from build123d import *

# Parameters (mm, degrees)
SKETCH1_W           = 103
SKETCH1_H           = 115
BOSS_EXTRUDE2_DEPTH = 20
SKETCH3_W           = 21
SKETCH3_H           = 25
CUT_EXTRUDE1_DEPTH  = 10
CUT_EXTRUDE2_DEPTH  = 46


with BuildPart() as part:
    # Sketch1 → Boss-Extrude2 (new body)
    with BuildSketch(Plane.XY):
        with Locations((51.5, 57.5)):
            Rectangle(SKETCH1_W, SKETCH1_H)
    extrude(amount=BOSS_EXTRUDE2_DEPTH)

    # Sketch3 → Cut-Extrude1 (cut)
    with BuildSketch(Plane.XY.offset(20)):
        with Locations((20.5, 92.5)):
            Rectangle(SKETCH3_W, SKETCH3_H)
        with Locations((51.5, 92.5)):
            Rectangle(SKETCH3_W, SKETCH3_H)
        with Locations((82.5, 92.5)):
            Rectangle(SKETCH3_W, SKETCH3_H)
        Polygon((10, 70), (10, 54.37934433), (10, 45), (31, 45), (31, 70), align=None)
        with Locations((51.5, 57.5)):
            Rectangle(SKETCH3_W, SKETCH3_H)
        Polygon((10, 35), (10, 17.462651727), (10, 10), (31, 10), (31, 35), align=None)
        with Locations((51.5, 22.5)):
            Rectangle(SKETCH3_W, SKETCH3_H)
        with Locations((82.5, 22.5)):
            Rectangle(SKETCH3_W, SKETCH3_H)
        with Locations((82.5, 57.5)):
            Rectangle(SKETCH3_W, SKETCH3_H)
    extrude(amount=-CUT_EXTRUDE1_DEPTH, mode=Mode.SUBTRACT)

    # Sketch4 → Cut-Extrude2 (cut)
    with BuildSketch(Plane.XY.offset(20)):
        with BuildLine():
            Line((0, 105), (0, 115))
            Line((0, 115), (10, 115))
            ThreePointArc((10, 115), (2.928932188, 112.071067812), (0, 105))
        make_face()
        with BuildLine():
            Line((93, 115), (103, 115))
            Line((103, 115), (103, 105))
            ThreePointArc((103, 105), (100.071067812, 112.071067812), (93, 115))
        make_face()
        with BuildLine():
            Line((103, 10), (103, 0))
            Line((103, 0), (93, 0))
            ThreePointArc((93, 0), (100.071067812, 2.928932188), (103, 10))
        make_face()
        with BuildLine():
            Line((10, 0), (0, 0))
            Line((0, 0), (0, 10))
            ThreePointArc((0, 10), (2.928932188, 2.928932188), (10, 0))
        make_face()
    extrude(amount=-CUT_EXTRUDE2_DEPTH, mode=Mode.SUBTRACT)


solid = part.part
Can you work these out from the model? Positions are in its coordinate system, mm. A direction names the side the tool comes from. Give positions to 0.01 mm unless a question says otherwise; leave off trailing zeros. Loops run counter-clockwise (first coordinate to the right, second up) from the corner with the lowest first, then second, coordinate; pieces in that order, holes last. Notation, with made-up numbers: (5, 11) -> (11, 11) arc R25 cw to (11, 24) -> close; hole circle Ø5 at (0, 35). An arc over 180 degrees is marked (long way). Return JSON: item names as keys, results as strings.
Q1. We'd pull the mould along Y, two halves only. Please class faces 1 (the face through (62, 22, 15)), 2 (the face through (99.99, 2.85, 10.14)), 3 (the face through (51, 58, 0)): released by +Y, released by -Y, zero draft, split by the parting line, or undercut.
Checks:
{"face 1": "undercut", "face 2": "released by -Y", "face 3": "zero draft"}
Q2. I want a section at C-C, the plane x = 56. List the corners of the cut face in (y, z) for me, then the cut area to 3 significant figures.
Checks:
{"outline": "(0, 0) -> (115, 0) -> (115, 20) -> (105, 20) -> (105, 10) -> (80, 10) -> (80, 20) -> (70, 20) -> (70, 10) -> (45, 10) -> (45, 20) -> (35, 20) -> (35, 10) -> (10, 10) -> (10, 20) -> (0, 20) -> close", "area": "1,550 mm2"}
Q3. I want a section at A-A, the plane y = 55.5. List the corners of the cut face in (x, z) for me, then the cut area to 3 significant figures.
Checks:
{"outline": "(0, 0) -> (103, 0) -> (103, 20) -> (93, 20) -> (93, 10) -> (72, 10) -> (72, 20) -> (62, 20) -> (62, 10) -> (41, 10) -> (41, 20) -> (31, 20) -> (31, 10) -> (10, 10) -> (10, 20) -> (0, 20) -> close", "area": "1,430 mm2"}
Q4. I need wall thicknesses on probe 1 along Y at (x, z) = (24, 10.75); probe 2 along X at (y, z) = (66.5, 18.25); probe 3 along Z at (x, y) = (92.5, 63). Which ranges of each line are inside material? Lowest first, please.
Checks:
{"probe 1": "y = 0 to 10, 35 to 45, 70 to 80, 105 to 115", "probe 2": "x = 0 to 10, 31 to 41, 62 to 72, 93 to 103", "probe 3": "z = 0 to 10"}
Q5. I want a section at B-B, the plane z = 13.25. Count the separate pieces of the cut face and the enclosed holes in it, then the cut area to 3 significant figures.
Checks:
{"separate pieces": "1", "enclosed holes": "9", "area": "7,030 mm2"}
Q6. On a 3-axis mill with a long thin cutter (end or side, diameter ignored), from which of +Z, -Z, +X, -X, +Y, -Y can I reach the whole of each face in a straight line? I mean faces 4 (the face through (10, 92, 15)), 5 (the face through (0, 57, 10)). Say none if no direction works.
Checks:
{"face 4": "+Z", "face 5": "+Z, -Z, -X, +Y, -Y"}
Q7. For pin 1 Ø10 at (x, y) = (52, 52) entering from +Z, with a flat end and sliding along its axis, tell me the tip position at first contact or that it passes through.
Checks:
{"pin 1": "stops at z = 10"}
